Autodesk Inventor part; units mm, degrees
ref_plane "YZ Plane" through (0, 0, 0) normal (1, 0, 0) x (0, 1, 0)
ref_plane "XZ Plane" through (0, 0, 0) normal (0, 1, 0) x (-1, 0, 0)
ref_plane "XY Plane" through (0, 0, 0) normal (0, 0, 1) x (1, 0, 0)
sketch "Sketch8" plane through (0, 0, 0) normal (0, 1, 0) x (-1, 0, 0)
  circle A0 centre (0, 0) radius 4.25
  line L0 (-1.5588, -2.7) -> (-3.1177, 0)
  line L1 (-3.1177, 0) -> (-1.5588, 2.7)
  line L2 (-1.5588, 2.7) -> (1.5588, 2.7)
  line L3 (1.5588, 2.7) -> (3.1177, 0)
  line L4 (3.1177, 0) -> (1.5588, -2.7)
  line L5 (1.5588, -2.7) -> (-1.5588, -2.7)
  line L6 (-5.95, 0) -> (5.95, 0)
  dimension "d57" = 8.5
  dimension "d58" = 5.4
extrude "Extrusion7" add sketch "Sketch8" along normal blind 4 contours L6 L3 L2 L1 A0 | A0 L6 L0 L5 L4
sketch "Sketch9" plane through (0, 4, 0) normal (0, 1, 0) x (1, 0, 0)
  circle A0 centre (0, 0) radius 4.25
  line L0 (-3.1177, 0) -> (-1.5588, 2.7)
  line L1 (-1.5588, 2.7) -> (1.5588, 2.7)
  line L2 (1.5588, 2.7) -> (3.1177, 0)
  line L3 (3.1177, 0) -> (1.5588, -2.7)
  line L4 (1.5588, -2.7) -> (-1.5588, -2.7)
  line L5 (-1.5588, -2.7) -> (-3.1177, 0)
  circle A1 centre (0, 0) radius 2.55
  dimension "d61" = 5.1
extrude "Extrusion8" add sketch "Sketch9" along normal blind 50 contours A0 | L0 L1 L2 L3 L4 L5
sketch "Sketch11" plane through (0, 0, 0) normal (0, -1, 0) x (1, 0, 0)
  circle A0 centre (0, 0) radius 4.25
  circle A1 centre (0, 0) radius 10
  dimension "d71" = 20
extrude "Extrusion10" add sketch "Sketch11" against normal blind 10
sketch "Sketch12" plane through (-1.5588, 0, -2.7) normal (0, 0, 1) x (1, 0, 0)
  line L0 (0, 0) -> (0, 4)
  line L1 (4.6765, 0) -> (4.6765, 4)
  circle A0 centre (1.5588, 2.3184) radius 1.4
  point P0 (1.5588, 0)
  dimension "d74" = 2.8
extrude "Extrusion11" cut sketch "Sketch12" along normal through all both and the other way through all
pattern_circular "Circular Pattern5" count 6 over 360 about axis through (0, 0, 0) along (0, 1, 0) of "Extrusion11"
properties part number "30_Cube_Z_Focus_MGN_NEMA_Motorcoupling_Captive_v3"
Geometry: final body of the model. Coordinates: model frame, mm. A direction names the side the tool comes from. Round coordinates to 2 decimals unless told otherwise and drop trailing zeros. Loops run counter-clockwise (first coordinate to the right, second up) from the corner with the lowest first, then second, coordinate; pieces in that order, holes last.
Q1. Pull-direction query (Y, two-part tool) for faces 1 (the cylindrical face through (-5.3, 0.95, 3.41)), 2 (the cylindrical face through (4.054, 31.692, 1.277)), 3 (the flat face through (4, 10, -2)), 4 (the cylindrical face through (4.88, 3.17, 4.1)); classes: released by +Y, released by -Y, zero draft, split by the parting line, or undercut.
Q2. Material intervals for L1, parallel to Z at x = 0, y = 15; L2, parallel to Y at x = 0, z = -8; L3, parallel to X at y = 38, z = -0.5, sorted ascending.
Q3. Pin query (flat end, axial travel): P1, Ø8, axis at x = 7.5, y = 14.5, coming from the -Z side; P2, Ø1.5, axis at y = 32.5, z = -3.5, coming from the +X side; P3, Ø10, axis at y = 26, z = 5, coming from the -X side; P4, Ø1.7, axis at x = 0, y = 2.32, coming from the +Z side. Return the tip coordinate at first contact, or that it passes through.
Q4. Section C-C on z = 8.5. Return loops of the section in (x, y).
Q5. Section D-D on z = -9. Return loops of the section in (x, y).
Q6. Access query for faces 5 (the flat face through (-1, 1, -2.7)), 6 (the flat face through (2.35, 0.64, 1.33)), 7 (the cylindrical face through (-0.3, 0.95, -6.3)). Directions: +Z, -Z, +X, -X, +Y, -Y. A direction counts if a zero-diameter tool reaches every point of the face in a straight line with its end or side. Return the directions, or none.
Q7. Section B-B on y = 9.5. Return loops of the section in (x, z), plus the area to 3 significant figures.
Q8. Section A-A on x = 0. Return loops of the section in (y, z).
Evaluation:
1. face 1: undercut
1. face 2: zero draft
1. face 3: released by +Y
1. face 4: undercut
2. L1: z = -4.25 to -2.55, 2.55 to 4.25
2. L2: y = 0 to 0.92, 3.72 to 10
2. L3: x = -4.22 to -2.5, 2.5 to 4.22
3. P1: stops at z = -2.41
3. P2: stops at x = 3.24
3. P3: stops at x = -4.25
3. P4: passes through
4. outline: (-5.27, 0) - (5.27, 0) - (5.27, 10) - (-5.27, 10) - close; hole circle Ø2.8 at (0, 2.32)
5. outline: (-4.36, 0) - (4.36, 0) - (4.36, 10) - (-4.36, 10) - close; hole circle Ø2.8 at (0, 2.32)
6. face 5: -Y
6. face 6: none
6. face 7: +Z, -Z
7. outline: circle Ø20 at (0, 0); hole circle Ø5.1 at (0, 0)
7. area: 294 mm2
8. outline: (0, -10) - (0.92, -10) - (0.92, -2.7) - (0, -2.7) - close; (0, 2.7) - (0.92, 2.7) - (0.92, 10) - (0, 10) - close; (3.72, -10) - (10, -10) - (10, -4.25) - (54, -4.25) - (54, -2.55) - (4, -2.55) - (4, -2.7) - (3.72, -2.7) - close; (3.72, 2.7) - (4, 2.7) - (4, 2.55) - (54, 2.55) - (54, 4.25) - (10, 4.25) - (10, 10) - (3.72, 10) - close
